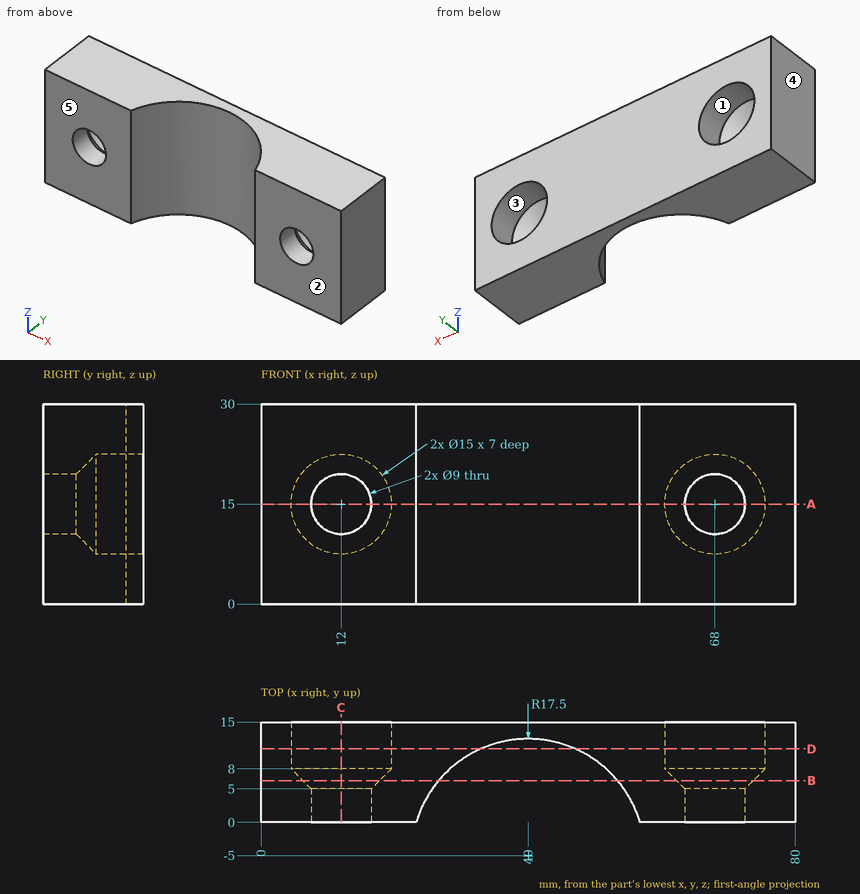
Check sheet for the drawn part. Datum: minimum x, y, z corner. Units: mm. A direction names the side the tool comes from. Give positions to 0.01 mm unless a question says otherwise; leave off trailing zeros. Loops run counter-clockwise (first coordinate to the right, second up) from the corner with the lowest first, then second, coordinate; pieces in that order, holes last.
1) Thickness scan on line 1 along Z through (x, y) = (68, 2.2); line 2 along Z through (x, y) = (12, 13.25); line 3 along X through (y, z) = (3.25, 15). Record the ranges inside material, lowest first.
2) Draft check along X on the marked faces 3, 4 and 5. Enter one of: pulls with the +X half, pulls with the -X half, needs draft (parallel to the pull), parting line crosses it, or undercut.
3) Sectioned sample at D-D, the plane y = 11. Enter the section's corners in (x, z), then the cut area to 3 significant figures.
4) Sectioned sample at C-C, the plane x = 12. Enter the section's corners in (y, z).
5) Sectioned sample at B-B, the plane y = 6.25. Enter the section's corners in (x, z).
6) Set-up check for the marked faces 1 and 2: record each of +Z, -Z, +X, -X, +Y, -Y from which the full face is reachable in a straight line by a thin tool's end or side.
7) Depth check by flat-ended pin: pin 1 Ø8 at (x, y) = (43.5, 4.5) entering from +Z (3 decimals); pin 2 Ø11.5 at (x, z) = (12, 15) entering from +Y. Enter the tip coordinate at first touch or a pass-through.
8) Sectioned sample at A-A, the plane z = 15. Enter the section's corners in (x, y), then the cut area to 3 significant figures.
Answers:
1. line 1: z = 0 to 10.5, 19.5 to 30
1. line 2: z = 0 to 7.5, 22.5 to 30
1. line 3: x = 0 to 7.5, 16.5 to 24.57, 55.43 to 63.5, 72.5 to 80
2. face 3: undercut
2. face 4: pulls with the -X half
2. face 5: needs draft
3. outline: (0, 0) - (32.91, 0) - (32.91, 30) - (0, 30) - close; (47.09, 0) - (80, 0) - (80, 30) - (47.09, 30) - close; hole circle Ø15 at (12, 15); hole circle Ø15 at (68, 15)
3. area: 1,620 mm2
4. outline: (0, 0) - (15, 0) - (15, 7.5) - (8, 7.5) - (5, 10.5) - (0, 10.5) - close; (0, 19.5) - (5, 19.5) - (8, 22.5) - (15, 22.5) - (15, 30) - (0, 30) - close
5. outline: (0, 0) - (26.6, 0) - (26.6, 30) - (0, 30) - close; (53.4, 0) - (80, 0) - (80, 30) - (53.4, 30) - close; hole circle Ø11.5 at (12, 15); hole circle Ø11.5 at (68, 15)
6. face 1: +Y
6. face 2: +Z, -Z, +X, -X, -Y
7. pin 1: passes through
7. pin 2: stops at y = 6.25
8. outline: (0, 0) - (7.5, 0) - (7.5, 5) - (4.5, 8) - (4.5, 15) - (0, 15) - close; (16.5, 0) - (23.23, 0) arc R17.5 cw to (56.77, 0) - (63.5, 0) - (63.5, 5) - (60.5, 8) - (60.5, 15) - (19.5, 15) - (19.5, 8) - (16.5, 5) - close; (72.5, 0) - (80, 0) - (80, 15) - (75.5, 15) - (75.5, 8) - (72.5, 5) - close
8. area: 520 mm2
